The drawing under review shows one solid part. Ordinate dimensions are in mm from its lowest x, y, z. A direction names the side the tool comes from. Round coordinates to 2 decimals unless told otherwise and drop trailing zeros. Order: outer loops, then holes, each group sorted by start corner. A loop starts at its lowest first (then second) coordinate and runs counter-clockwise, first axis right, second up. Notation, with made-up numbers: M -20.5,-8.5 L 28.5,-8.5 A25 cw 28.5,15.5 Z; hole C 26,52 d5. An arc over 180 degrees is marked long. Answer as a JSON object with one key per item and string values. Group by question number.
1) Consider section D-D, the plane y = 16.75. Write out the cut boundary in (x, z), then the cut area to 3 significant figures.
2) Consider section C-C, the plane z = 5.5. Write out the cut boundary in (x, y).
3) For the marked faces 5, 6, 7, 8 and 9, list the 3-axis set-ups (+Z, -Z, +X, -X, +Y, -Y) from which the entire face can be reached by the end or side of a thin tool; tool diameter is ignored.
4) Consider section A-A, the plane y = 3. Write out the cut boundary in (x, z).
5) The part is to be moulded in two halves that separate along X. For the marked faces 1, 2, 3 and 4, say which applies: +X half, -X half, draft (parallel to the pull), parting line (faces both ways), or undercut.
6) Insertion check: pin 1 Ø10 at (x, y) = (52, 16.5) entering from +Z; pin 2 Ø12 at (x, y) = (8, 11.5) entering from -Z; pin 3 Ø4 at (y, z) = (3.5, 25) entering from -X. Each pin has a flat end and moves straight along its axis. Give the tip position at first contact, or say it passes through.
7) Consider section B-B, the plane x = 32. Write out the cut boundary in (y, z), then the cut area to 3 significant figures.
8) To check wall thickness, follow line 1 (Y direction, x = 36.5, z = 29); line 2 (X direction, y = 19.25, z = 21.5); line 3 (X direction, y = 16.25, z = 3). State the ranges of each line that lie inside material, in increasing order.
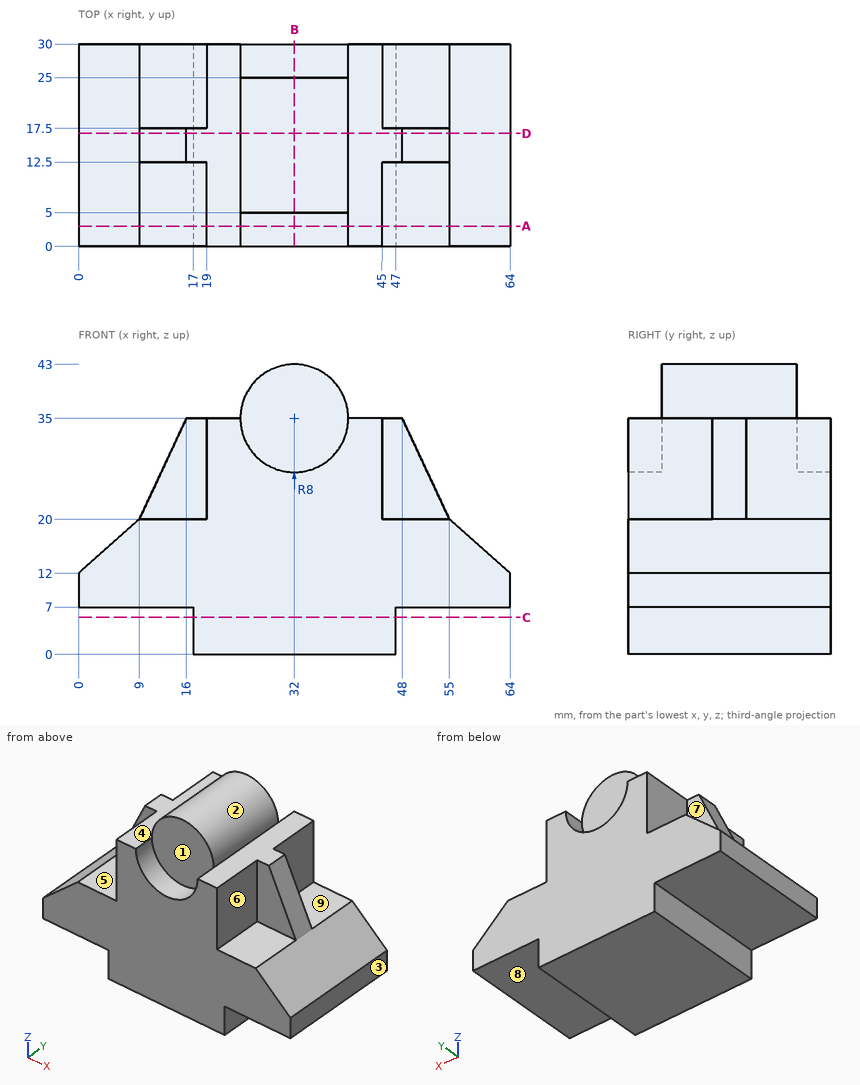
Results list:
{
 "1": {"outline": "M 0,7 L 17,7 L 17,0 L 47,0 L 47,7 L 64,7 L 64,12 L 55,20 L 48,35 L 40,35 A8 ccw 24,35 L 16,35 L 9,20 L 0,12 Z", "area": "1,660 mm^2"},
 "2": {"outline": "M 17,0 L 47,0 L 47,30 L 17,30 Z"},
 "3": {"face 5": "+Z, -X, -Y", "face 6": "+Z, +X, -Y", "face 7": "+Z, -X, +Y", "face 8": "-Z, +X, +Y, -Y", "face 9": "+Z, +X, +Y"},
 "4": {"outline": "M 0,7 L 17,7 L 17,0 L 47,0 L 47,7 L 64,7 L 64,12 L 55,20 L 45,20 L 45,35 L 40,35 A8 cw 24,35 L 19,35 L 19,20 L 9,20 L 0,12 Z"},
 "5": {"face 1": "undercut", "face 2": "parting line", "face 3": "+X half", "face 4": "draft"},
 "6": {"pin 1": "z = 35", "pin 2": "z = 7", "pin 3": "x = 19"},
 "7": {"outline": "M 0,0 L 30,0 L 30,27 L 25,27 L 25,43 L 5,43 L 5,27 L 0,27 Z", "area": "1,130 mm^2"},
 "8": {"line 1": "5 to 25", "line 2": "19 to 45", "line 3": "17 to 47"}
}
